Part model, mm, in its own coordinate system. A direction names the side the tool comes from. Give positions to 0.01 mm unless a question says otherwise; leave off trailing zeros. Order: outer loops, then holes, each group sorted by start corner. A loop starts at its lowest first (then second) coordinate and runs counter-clockwise, first axis right, second up. Notation, with made-up numbers: (-38, 40) - (-32, 40) arc R34 ccw to (-32, 73) - close; hole circle Ø3 at (-10, 63.25). An arc over 180 degrees is marked (long way). One line per item, written item: value.
```python
from build123d import *

# Parameters (mm, degrees)
BOSS_EXTRUDE2_DEPTH = 28
SKETCH3_W           = 40
SKETCH3_H           = 38
BOSS_EXTRUDE3_DEPTH = 10
CUT_EXTRUDE2_DEPTH  = 8
SKETCH6_W           = 20.7
SKETCH6_H           = 38
CUT_EXTRUDE3_DEPTH  = 43
CUT_EXTRUDE4_DEPTH  = 43
BOSS_EXTRUDE5_DEPTH = 8
SKETCH10_R          = 10
BOSS_EXTRUDE6_DEPTH = 4
SKETCH11_R          = 8
CUT_EXTRUDE5_DEPTH  = 4
SKETCH12_R          = 8
CUT_EXTRUDE6_DEPTH  = 10
SKETCH13_W          = 3.3
SKETCH13_H          = 31.65
CUT_EXTRUDE7_DEPTH  = 10
SKETCH14_W          = 3.3
SKETCH14_H          = 31.65
CUT_EXTRUDE8_DEPTH  = 10
SKETCH15_W          = 16.679991472
SKETCH15_H          = 28
CUT_EXTRUDE9_DEPTH  = 253
SKETCH16_W          = 10.1
SKETCH16_H          = 7
CUT_EXTRUDE11_DEPTH = 13
SKETCH17_W          = 2.35
SKETCH17_H          = 11.05285785
BOSS_EXTRUDE7_DEPTH = 3


with BuildPart() as part:
    # Sketch1 → Boss-Extrude2 (new body)
    with BuildSketch(Plane(origin=(0, 0, 0), x_dir=(1, 0, 0), z_dir=(0, 1, 0))):
        Polygon((40, -2), (40, -40), (0, -40), (0, -2), (2.35, -2), (2.35, -2.35), (2.35, -20), (2.35, -37.65), (37.65, -37.65), (37.65, -20), (37.65, -2.35), (37.65, -2), align=None)
    extrude(amount=BOSS_EXTRUDE2_DEPTH)

    # Sketch3 → Boss-Extrude3 (add)
    with BuildSketch(Plane.XZ):
        with Locations((20, 21)):
            Rectangle(SKETCH3_W, SKETCH3_H)
    extrude(amount=BOSS_EXTRUDE3_DEPTH)

    # Sketch5 → Cut-Extrude2 (cut)
    with BuildSketch(Plane(origin=(0, 0, 0), x_dir=(1, 0, 0), z_dir=(0, 1, 0))):
        Polygon((9.65, -20), (9.65, -57.9), (20, -57.9), (30.35, -57.9), (30.35, -20), (30.35, -2), (9.65, -2), align=None)
    extrude(amount=-CUT_EXTRUDE2_DEPTH, mode=Mode.SUBTRACT)

    # Sketch6 → Cut-Extrude3 (cut)
    with BuildSketch(Plane(origin=(0, -8, 0), x_dir=(1, 0, 0), z_dir=(0, 1, 0))):
        with Locations((20, -21)):
            Rectangle(SKETCH6_W, SKETCH6_H)
    extrude(amount=CUT_EXTRUDE3_DEPTH, mode=Mode.SUBTRACT)

    # Sketch7 → Cut-Extrude4 (cut)
    with BuildSketch(Plane(origin=(0, -8, 0), x_dir=(1, 0, 0), z_dir=(0, 1, 0))):
        Polygon((20, -4), (18, -4), (18, -2), (22, -2), (22, -4), align=None)
    extrude(amount=-CUT_EXTRUDE4_DEPTH, mode=Mode.SUBTRACT)

    # Sketch9 → Boss-Extrude5 (add)
    with BuildSketch(Plane.XZ.offset(10)):
        Polygon((30.1, 44.2), (30.1, 40), (32.1, 40), (32.1, 46.2), (18, 46.2), (9.9, 46.2), (7.9, 46.2), (7.9, 40), (9.9, 40), (9.9, 44.2), align=None)
    extrude(amount=-BOSS_EXTRUDE5_DEPTH)

    # Sketch10 → Boss-Extrude6 (add)
    with BuildSketch(Plane.XZ.offset(10)):
        with Locations(Location((20, 20, 0), (0, 0, 270))):
            Circle(SKETCH10_R)
    extrude(amount=BOSS_EXTRUDE6_DEPTH)

    # Sketch11 → Cut-Extrude5 (cut)
    with BuildSketch(Plane(origin=(0, -14, 0), x_dir=(-1, 0, 0), z_dir=(0, -1, 0))):
        with Locations(Location((-20, -20, 0), (0, 0, 90))):
            Circle(SKETCH11_R)
    extrude(amount=-CUT_EXTRUDE5_DEPTH, mode=Mode.SUBTRACT)

    # Sketch12 → Cut-Extrude6 (cut)
    with BuildSketch(Plane.XZ.offset(10)):
        with Locations(Location((20, 20, 0), (0, 0, 270))):
            Circle(SKETCH12_R)
    extrude(amount=-CUT_EXTRUDE6_DEPTH, mode=Mode.SUBTRACT)

    # Sketch13 → Cut-Extrude7 (cut)
    with BuildSketch(Plane(origin=(0, 0, 0), x_dir=(1, 0, 0), z_dir=(0, 1, 0))):
        with Locations((6, -19.825)):
            Rectangle(SKETCH13_W, SKETCH13_H)
    extrude(amount=-CUT_EXTRUDE7_DEPTH, mode=Mode.SUBTRACT)

    # Sketch14 → Cut-Extrude8 (cut)
    with BuildSketch(Plane(origin=(0, 0, 0), x_dir=(1, 0, 0), z_dir=(0, 1, 0))):
        with Locations((34, -19.825)):
            Rectangle(SKETCH14_W, SKETCH14_H)
    extrude(amount=-CUT_EXTRUDE8_DEPTH, mode=Mode.SUBTRACT)

    # Sketch15 → Cut-Extrude9 (cut)
    with BuildSketch(Plane(origin=(40, 0, 0), x_dir=(0, 0, -1), z_dir=(1, 0, 0))):
        with Locations((-21.392853586, 14)):
            Rectangle(SKETCH15_W, SKETCH15_H)
    extrude(amount=-CUT_EXTRUDE9_DEPTH, mode=Mode.SUBTRACT)

    # Sketch16 → Cut-Extrude11 (cut)
    with BuildSketch(Plane.XZ.offset(10)):
        with Locations((20, 36.5)):
            Rectangle(SKETCH16_W, SKETCH16_H)
    extrude(amount=-CUT_EXTRUDE11_DEPTH, mode=Mode.SUBTRACT)

    # Sketch17 → Boss-Extrude7 (add)
    with BuildSketch(Plane(origin=(0, 28, 0), x_dir=(1, 0, 0), z_dir=(0, 1, 0))):
        Polygon((40, -40), (40, -29.732849322), (37.65, -29.732849322), (37.65, -37.65), (30.35, -37.65), (30.35, -40), align=None)
        Polygon((9.65, -40), (0, -40), (0, -29.732849322), (2.35, -29.732849322), (2.35, -37.65), (9.65, -37.65), align=None)
        with Locations((1.175, -7.526428925)):
            Rectangle(SKETCH17_W, SKETCH17_H)
        with Locations((38.825, -7.526428925)):
            Rectangle(SKETCH17_W, SKETCH17_H)
    extrude(amount=BOSS_EXTRUDE7_DEPTH)


solid = part.part
```
1) Drill centre lines: line 1 along X through (y, z) = (-9, 20); line 2 along X through (y, z) = (16.5, 11); line 3 along X through (y, z) = (-7, 25). Where is each one in solid material? Low to high. Write a range as from..to.
Outcome:
line 1: x = 0..4.35, 7.65..12, 28..32.35, 35.65..40
line 2: x = 0..2.35, 37.65..40
line 3: x = 0..4.35, 7.65..9.65, 30.35..32.35, 35.65..40
2) Pin check, flat tips, straight feed: pin 1 (3 mm diameter, centred on y = -7, z = 44, fed in from -X); pin 2 (10 mm diameter, centred on x = 28, y = 9, fed in from -Z); pin 3 (6 mm diameter, centred on x = 31, z = 12.5, fed in from +Y). Stop position of each tip, or through.
Outcome:
pin 1: stops at x = 7.9
pin 2: stops at z = 37.65
pin 3: stops at y = 0
3) Mould opens along Z. For faces 1 (the flat face through (22, -8, 12)), 2 (the flat face through (34, 15, 37.65)), 3 (the flat face through (34, -5, 35.65)) say: released by +Z, released by -Z, zero draft, split by the parting line, or undercut.
Outcome:
face 1: zero draft
face 2: released by -Z
face 3: undercut
4) Cut at D-D, the plane z = 41.5. Give the cut face in (x, y), then the cut area to 3 significant figures.
Outcome:
outline: (7.9, -10) - (9.9, -10) - (9.9, -2) - (7.9, -2) - close; (30.1, -10) - (32.1, -10) - (32.1, -2) - (30.1, -2) - close
area: 32.0 mm^2
5) Cut at B-B, the plane z = 20. Give the cut face in (x, y).
Outcome:
outline: (0, -10) - (4.35, -10) - (4.35, 0) - (0, 0) - close; (7.65, -10) - (10, -10) - (10, -14) - (12, -14) - (12, -8) - (9.65, -8) - (9.65, 0) - (7.65, 0) - close; (28, -14) - (30, -14) - (30, -10) - (32.35, -10) - (32.35, 0) - (30.35, 0) - (30.35, -8) - (28, -8) - close; (35.65, -10) - (40, -10) - (40, 0) - (35.65, 0) - close
6) Cut at C-C, the plane x = 20. Give the cut face in (y, z), then the cut area to 3 significant figures.
Outcome:
outline: (-14, 10) - (-10, 10) - (-10, 4) - (-8, 4) - (-8, 12) - (-14, 12) - close; (-14, 28) - (-8, 28) - (-8, 33) - (-10, 33) - (-10, 30) - (-14, 30) - close; (-10, 44.2) - (-2, 44.2) - (-2, 46.2) - (-10, 46.2) - close
area: 58.0 mm^2
7) Cut at A-A, the plane x = 34. Give the cut face in (y, z).
Outcome:
outline: (-10, 2) - (0, 2) - (0, 4) - (-10, 4) - close; (-10, 35.65) - (0, 35.65) - (0, 37.65) - (31, 37.65) - (31, 40) - (-10, 40) - close
8) Which spindle directions (+Z, -Z, +X, -X, +Y, -Y) get a long thin tool onto all of the face, cutting with end or side? Do faces 4 (the cylindrical face through (23, -11.97, 10.46)), 5 (the flat face through (12, -9, 40)), 6 (the flat face through (39, 15, 29.733)), 7 (the flat face through (30.35, -2, 24)), 8 (the flat face through (2, 31, 37)). Say none if no direction does.
Outcome:
face 4: -Y
face 5: +Y, -Y
face 6: +X, -X, +Y
face 7: -Z, +Y
face 8: +Z, -Z, +X, -X, +Y
